For this review, take the finished solid that the model builds, in its own axes (mm). Face numbers are marked on the shaded views. Round coordinates to 2 decimals unless told otherwise and drop trailing zeros. Order: outer loops, then holes, each group sorted by start corner. A loop starts at its lowest first (then second) coordinate and runs counter-clockwise, first axis right, second up. Notation, with made-up numbers: (62.5, 82) - (102.5, 82) arc R11 cw to (102.5, 98) - close; hole circle Ø11 at (71, 32.5). An arc over 180 degrees is marked (long way). One line per question, with ' | ' between items.
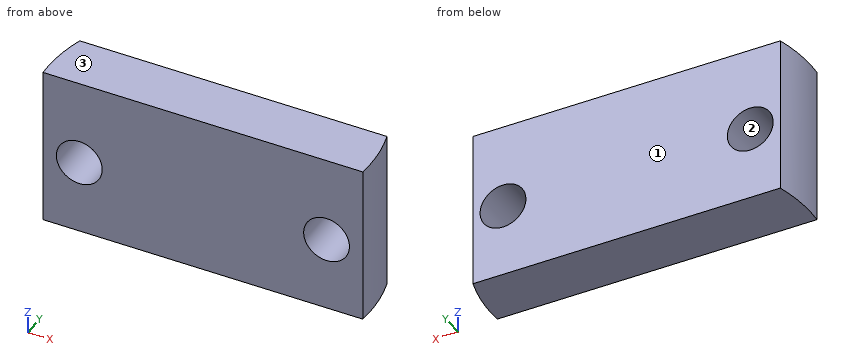
```python
from build123d import *

# Parameters (mm, degrees)
BOSS_EXTRUDE1_DEPTH = 15
SKETCH3_R           = 2
CUT_EXTRUDE1_DEPTH  = 22.117601772
CUT_EXTRUDE3_DEPTH  = 1


with BuildPart() as part:
    # Sketch2 → Boss-Extrude1 (new body)
    with BuildSketch(Plane.XY):
        with BuildLine():
            Line((0, 3.99956576), (-13.41495138, 3.99956576))
            ThreePointArc((-13.41495138, 3.99956576), (-13.915210617, 1.524585285), (-13.962716312, -1))
            Line((-13.962716312, -1), (0, -1))
            Line((0, -1), (13.962716312, -1))
            ThreePointArc((13.962716312, -1), (13.915210617, 1.524585285), (13.41495138, 3.99956576))
            Line((13.41495138, 3.99956576), (0, 3.99956576))
        make_face()
    extrude(amount=BOSS_EXTRUDE1_DEPTH)

    # Sketch3 → Cut-Extrude1 (cut, through all)
    with BuildSketch(Plane(origin=(0, 3.99956576, 0), x_dir=(1, 0, 0), z_dir=(0, 1, 0))):
        with Locations(Location((10.795, -7.5, 0), (0, 0, 270))):
            Circle(SKETCH3_R)
        with Locations(Location((-10.795, -7.5, 0), (0, 0, 90))):
            Circle(SKETCH3_R)
    extrude(amount=-CUT_EXTRUDE1_DEPTH, mode=Mode.SUBTRACT)

    # Sketch4 → Cut-Extrude3 (cut)
    with BuildSketch(Plane.XY):
        with BuildLine():
            Line((13.962716312, -1), (-13.962716312, -1))
            ThreePointArc((-13.962716312, -1), (-13.915210617, 1.524585285), (-13.41495138, 3.99956576))
            Line((-13.41495138, 3.99956576), (0, 3.99956576))
            Line((0, 3.99956576), (13.41495138, 3.99956576))
            ThreePointArc((13.41495138, 3.99956576), (13.915210617, 1.524585285), (13.962716312, -1))
        make_face()
    extrude(amount=CUT_EXTRUDE3_DEPTH, mode=Mode.SUBTRACT)


solid = part.part
```
(1) We need section B-B on y = 0. State the section outline as (x, z) points (3 decimals).
Output values:
outline: (-13.998, 1) - (13.998, 1) - (13.998, 15) - (-13.998, 15) - close; hole circle Ø4 at (-10.795, 7.5); hole circle Ø4 at (10.795, 7.5)
(2) Insertion check: pin 1 (1.5 mm diameter, centred on y = 2.5, z = 12.5, fed in from -X); pin 2 (1.5 mm diameter, centred on y = 1, z = 5, fed in from -X). Each pin has a flat end and moves straight along its axis. Give the tip position at first contact, or say it passes through.
Output values:
pin 1: x = -13.89 | pin 2: x = -14
(3) For probe 1 along X at (y, z) = (2.75, 7.5) (3 decimals); probe 2 along X at (y, z) = (2.4, 7.5) (3 decimals); probe 3 along X at (y, z) = (0.35, 2.5), list the stretches that pass through material, from the lowest coordinate up. Write a range as [from, to].
Output values:
probe 1: [-13.726, -12.795], [-8.795, 8.795], [12.795, 13.726] | probe 2: [-13.791, -12.795], [-8.795, 8.795], [12.795, 13.791] | probe 3: [-13.99, 13.99]
(4) Mouldability with a two-part tool opening along Z and no side actions: class the marked faces 1, 2 and 3 as released by +Z, released by -Z, zero draft, split by the parting line, or undercut.
Output values:
face 1: zero draft | face 2: undercut | face 3: released by +Z
(5) We need section A-A on z = 7.5. State the section outline as (x, y) points (3 decimals), plus the area to 3 significant figures.
Output values:
outline: (-13.963, -1) - (-12.795, -1) - (-12.795, 4) - (-13.415, 4) arc R13.998 ccw to start; (-8.795, -1) - (8.795, -1) - (8.795, 4) - (-8.795, 4) - close; (12.795, -1) - (13.963, -1) arc R13.998 ccw to (13.415, 4) - (12.795, 4) - close | area: 98.4 mm^2
(6) We need section C-C on z = 6. State the section outline as (x, y) points.
Output values:
outline: (-13.96, -1) - (-12.12, -1) - (-12.12, 4) - (-13.41, 4) arc R14 ccw to start; (-9.47, -1) - (9.47, -1) - (9.47, 4) - (-9.47, 4) - close; (12.12, -1) - (13.96, -1) arc R14 ccw to (13.41, 4) - (12.12, 4) - close
